Source: CAD feature listing. Evaluate the final solid. Frame: model axes, mm. A direction names the side the tool comes from. Round coordinates to 2 decimals unless told otherwise and drop trailing zeros. Order: outer loops, then holes, each group sorted by start corner. A loop starts at its lowest first (then second) coordinate and runs counter-clockwise, first axis right, second up. Notation, with made-up numbers: (70, -38) -> (114, -38) arc R19 ccw to (114, -32) -> close; hole circle Ø11 at (-21, 36.25). An arc over 180 degrees is marked (long way). Write item = value, one per line. Start each with the question number.
(1) Cut plane D-D on z = -25. Return the cut outline in (x, y).
(2) Cut plane A-A on y = 0. Return the cut outline in (x, z).
(3) Ray query, line 1 (Y direction, x = 3.3, z = 0); line 2 (Y direction, x = 3.6, z = 23); line 3 (Z direction, x = 4.2, y = -25). Return the intervals inside material, ascending.
(4) Cut plane C-C on x = 2.5. Give the number of separate pieces and of enclosed holes in the cut face, then the cut area to 3 significant figures.
(5) Contact query for flat-ended pins moving along their axis: pin 1 Ø1.5 at (x, z) = (1.5, -17.5) entering from -Y; pin 2 Ø2.5 at (x, z) = (3, 24.5) entering from +Y. Output: stop coordinate, or through.
(6) Draft query along Z for faces 5 (the face through (2, 0, -60)), 6 (the face through (2, 30, -53)), 7 (the face through (3, -33, -7.5)). Return one class per face: released by +Z, released by -Z, zero draft, split by the parting line, or undercut.
(7) Reachability of faces 1 (the face through (2, -30, 53)), 2 (the face through (2.54, -27.24, 45.96)), 3 (the face through (3, 26, -22.1)), 4 (the face through (3, -33, 7.5)) from +Z, -Z, +X, -X, +Y, -Y: full face, straight path, thin tool, end or side. Return the list, or none.
(8) Cut plane B-B on z = 0. Return the cut outline in (x, y).
from build123d import *

# Parameters (mm, degrees)
SKETCH_1_W          = 120
SKETCH_1_H          = 60
EXTRUDE_1_DEPTH     = 5
SKETCH_2_R          = 8
CUT_EXTRUDE_1_DEPTH = 5
SKETCH_3_W          = 15
SKETCH_3_H          = 5
EXTRUDE_2_DEPTH     = 5
CUT_EXTRUDE_2_DEPTH = 5
CUT_EXTRUDE_3_DEPTH = 10
FILLET_1_R          = 3
CUT_EXTRUDE_4_DEPTH = 10
FILLET_2_R          = 2


with BuildPart() as part:
    # 草图1 → 凸台-拉伸1 (new body)
    with BuildSketch(Plane(origin=(0, 0, 0), x_dir=(0, 0, -1), z_dir=(1, 0, 0))):
        Rectangle(SKETCH_1_W, SKETCH_1_H)
    extrude(amount=EXTRUDE_1_DEPTH)

    # 草图2 → 切除-拉伸1 (cut, symmetric)
    with BuildSketch(Plane(origin=(5, 0, 0), x_dir=(0, 0, -1), z_dir=(1, 0, 0))):
        Circle(SKETCH_2_R)
    extrude(amount=CUT_EXTRUDE_1_DEPTH, both=True, mode=Mode.SUBTRACT)

    # 草图3 → 凸台-拉伸2 (add)
    with BuildSketch(Plane(origin=(5, 0, 0), x_dir=(0, 0, -1), z_dir=(1, 0, 0))):
        with Locations((0, 32.5)):
            Rectangle(SKETCH_3_W, SKETCH_3_H)
        with Locations((-40, 32.5)):
            Rectangle(SKETCH_3_W, SKETCH_3_H)
        with Locations((40, 32.5)):
            Rectangle(SKETCH_3_W, SKETCH_3_H)
        with Locations((40, -32.5)):
            Rectangle(SKETCH_3_W, SKETCH_3_H)
        with Locations((-40, -32.5)):
            Rectangle(SKETCH_3_W, SKETCH_3_H)
        with Locations((0, -32.5)):
            Rectangle(SKETCH_3_W, SKETCH_3_H)
    extrude(amount=-EXTRUDE_2_DEPTH)

    # 草图4 → 切除-拉伸2 (cut)
    with BuildSketch(Plane(origin=(5, 0, 0), x_dir=(0, 0, -1), z_dir=(1, 0, 0))):
        Polygon((-22.1, 30), (-22.1, 22), (-23.5, 22), (-23.5, 15), (-16.5, 15), (-16.5, 22), (-17.9, 22), (-17.9, 30), align=None)
        Polygon((17.9, 30), (17.9, 22), (16.5, 22), (16.5, 15), (23.5, 15), (23.5, 22), (22.1, 22), (22.1, 30), align=None)
        Polygon((22.1, -30), (22.1, -22), (23.5, -22), (23.5, -15), (16.5, -15), (16.5, -22), (17.9, -22), (17.9, -30), align=None)
        Polygon((-17.9, -30), (-17.9, -22), (-16.5, -22), (-16.5, -15), (-23.5, -15), (-23.5, -22), (-22.1, -22), (-22.1, -30), align=None)
    extrude(amount=-CUT_EXTRUDE_2_DEPTH, mode=Mode.SUBTRACT)

    # 草图5 → 切除-拉伸3 (cut)
    with BuildSketch(Plane(origin=(5, 0, 0), x_dir=(0, 0, -1), z_dir=(1, 0, 0))):
        with BuildLine():
            Line((-46.321552745, 25.480053053), (-41.931231517, 9.173145635))
            ThreePointArc((-41.931231517, 9.173145635), (-40, 7.693092582), (-38.068768483, 9.173145635))
            Line((-38.068768483, 9.173145635), (-33.678447255, 25.480053053))
            ThreePointArc((-33.678447255, 25.480053053), (-34.022244696, 27.216574311), (-35.609678772, 28))
            Line((-35.609678772, 28), (-44.390321228, 28))
            ThreePointArc((-44.390321228, 28), (-45.977755304, 27.216574311), (-46.321552745, 25.480053053))
        make_face()
        with BuildLine():
            Line((-49.120413153, 22.331136171), (-41.994161638, 2.733944505))
            ThreePointArc((-41.994161638, 2.733944505), (-41.512509026, 0), (-41.994161638, -2.733944505))
            Line((-41.994161638, -2.733944505), (-49.120413153, -22.331136171))
            ThreePointArc((-49.120413153, -22.331136171), (-51.347005984, -23.617316729), (-53, -21.647650045))
            Line((-53, -21.647650045), (-53, 21.647650045))
            ThreePointArc((-53, 21.647650045), (-51.347005984, 23.617316729), (-49.120413153, 22.331136171))
        make_face()
        with BuildLine():
            Line((-38.068768483, -9.173145635), (-33.678447255, -25.480053053))
            ThreePointArc((-33.678447255, -25.480053053), (-34.022244696, -27.216574311), (-35.609678772, -28))
            Line((-35.609678772, -28), (-44.390321228, -28))
            ThreePointArc((-44.390321228, -28), (-45.977755304, -27.216574311), (-46.321552745, -25.480053053))
            Line((-46.321552745, -25.480053053), (-41.931231517, -9.173145635))
            ThreePointArc((-41.931231517, -9.173145635), (-40, -7.693092582), (-38.068768483, -9.173145635))
        make_face()
        with BuildLine():
            Line((-38.005838362, -2.733944505), (-30.879586847, -22.331136171))
            ThreePointArc((-30.879586847, -22.331136171), (-28.652994016, -23.617316729), (-27, -21.647650045))
            Line((-27, -21.647650045), (-27, 21.647650045))
            ThreePointArc((-27, 21.647650045), (-28.652994016, 23.617316729), (-30.879586847, 22.331136171))
            Line((-30.879586847, 22.331136171), (-38.005838362, 2.733944505))
            ThreePointArc((-38.005838362, 2.733944505), (-38.487490974, 0), (-38.005838362, -2.733944505))
        make_face()
        with BuildLine():
            Line((27, -21.647650045), (27, 21.647650045))
            ThreePointArc((27, 21.647650045), (28.652994016, 23.617316729), (30.879586847, 22.331136171))
            Line((30.879586847, 22.331136171), (38.005838362, 2.733944505))
            ThreePointArc((38.005838362, 2.733944505), (38.487490974, 0), (38.005838362, -2.733944505))
            Line((38.005838362, -2.733944505), (30.879586847, -22.331136171))
            ThreePointArc((30.879586847, -22.331136171), (28.652994016, -23.617316729), (27, -21.647650045))
        make_face()
        with BuildLine():
            Line((35.609678772, -28), (44.390321228, -28))
            ThreePointArc((44.390321228, -28), (45.977755304, -27.216574311), (46.321552745, -25.480053053))
            Line((46.321552745, -25.480053053), (41.931231517, -9.173145635))
            ThreePointArc((41.931231517, -9.173145635), (40, -7.693092582), (38.068768483, -9.173145635))
            Line((38.068768483, -9.173145635), (33.678447255, -25.480053053))
            ThreePointArc((33.678447255, -25.480053053), (34.022244696, -27.216574311), (35.609678772, -28))
        make_face()
        with BuildLine():
            Line((53, -21.647650045), (53, 21.647650045))
            ThreePointArc((53, 21.647650045), (51.347005984, 23.617316729), (49.120413153, 22.331136171))
            Line((49.120413153, 22.331136171), (41.994161638, 2.733944505))
            ThreePointArc((41.994161638, 2.733944505), (41.512509026, 0), (41.994161638, -2.733944505))
            Line((41.994161638, -2.733944505), (49.120413153, -22.331136171))
            ThreePointArc((49.120413153, -22.331136171), (51.347005984, -23.617316729), (53, -21.647650045))
        make_face()
        with BuildLine():
            Line((35.609678772, 28), (44.390321228, 28))
            ThreePointArc((44.390321228, 28), (45.977755304, 27.216574311), (46.321552745, 25.480053053))
            Line((46.321552745, 25.480053053), (41.931231517, 9.173145635))
            ThreePointArc((41.931231517, 9.173145635), (40, 7.693092582), (38.068768483, 9.173145635))
            Line((38.068768483, 9.173145635), (33.678447255, 25.480053053))
            ThreePointArc((33.678447255, 25.480053053), (34.022244696, 27.216574311), (35.609678772, 28))
        make_face()
    extrude(amount=-CUT_EXTRUDE_3_DEPTH, mode=Mode.SUBTRACT)

    # 圆角1
    fillet_1_edges = [part.edges().sort_by_distance(p)[0] for p in [
        (2.5, 30, 60),
        (2.5, 30, -60),
        (2.5, -30, -60),
        (2.5, -30, 60),
    ]]
    fillet(fillet_1_edges, radius=FILLET_1_R)

    # 草图6 → 切除-拉伸4 (cut)
    with BuildSketch(Plane(origin=(5, 0, 0), x_dir=(0, 0, -1), z_dir=(1, 0, 0))):
        with BuildLine():
            Line((-49.5, 30), (-47.5, 30))
            ThreePointArc((-47.5, 30), (-48.5, 29), (-49.5, 30))
        make_face()
        with BuildLine():
            Line((-32.5, 30), (-30.5, 30))
            ThreePointArc((-30.5, 30), (-31.5, 29), (-32.5, 30))
        make_face()
        with BuildLine():
            Line((-9.5, 30), (-7.5, 30))
            ThreePointArc((-7.5, 30), (-8.5, 29), (-9.5, 30))
        make_face()
        with BuildLine():
            Line((7.5, 30), (9.5, 30))
            ThreePointArc((9.5, 30), (8.5, 29), (7.5, 30))
        make_face()
        with BuildLine():
            Line((30.5, 30), (32.5, 30))
            ThreePointArc((32.5, 30), (31.5, 29), (30.5, 30))
        make_face()
        with BuildLine():
            Line((47.5, 30), (49.5, 30))
            ThreePointArc((49.5, 30), (48.5, 29), (47.5, 30))
        make_face()
        with BuildLine():
            Line((47.5, -30), (49.5, -30))
            ThreePointArc((49.5, -30), (48.5, -29), (47.5, -30))
        make_face()
        with BuildLine():
            Line((30.5, -30), (32.5, -30))
            ThreePointArc((32.5, -30), (31.5, -29), (30.5, -30))
        make_face()
        with BuildLine():
            Line((7.5, -30), (9.5, -30))
            ThreePointArc((9.5, -30), (8.5, -29), (7.5, -30))
        make_face()
        with BuildLine():
            Line((-9.5, -30), (-7.5, -30))
            ThreePointArc((-7.5, -30), (-8.5, -29), (-9.5, -30))
        make_face()
        with BuildLine():
            Line((-32.5, -30), (-30.5, -30))
            ThreePointArc((-30.5, -30), (-31.5, -29), (-32.5, -30))
        make_face()
        with BuildLine():
            Line((-49.5, -30), (-47.5, -30))
            ThreePointArc((-47.5, -30), (-48.5, -29), (-49.5, -30))
        make_face()
    extrude(amount=-CUT_EXTRUDE_4_DEPTH, mode=Mode.SUBTRACT)

    # 圆角2
    fillet_2_edges = [part.edges().sort_by_distance(p)[0] for p in [
        (2.5, -15, 23.5),
        (2.5, -15, 16.5),
        (2.5, -15, -16.5),
        (2.5, -15, -23.5),
        (2.5, 15, -23.5),
        (2.5, 15, -16.5),
        (2.5, 15, 16.5),
        (2.5, 15, 23.5),
    ]]
    fillet(fillet_2_edges, radius=FILLET_2_R)


solid = part.part
Evaluation:
q1.outline = (0, -30) -> (5, -30) -> (5, 30) -> (0, 30) -> close
q2.outline = (0, -60) -> (5, -60) -> (5, -53) -> (0, -53) -> close; (0, -41.51) -> (5, -41.51) -> (5, -38.49) -> (0, -38.49) -> close; (0, -27) -> (5, -27) -> (5, -8) -> (0, -8) -> close; (0, 8) -> (5, 8) -> (5, 27) -> (0, 27) -> close; (0, 38.49) -> (5, 38.49) -> (5, 41.51) -> (0, 41.51) -> close; (0, 53) -> (5, 53) -> (5, 60) -> (0, 60) -> close
q3.line_1 = -35 to -8, 8 to 35
q3.line_2 = -30 to -22, -15.68 to 15.68, 22 to 30
q3.line_3 = -60 to -46.19, -33.81 to -22.1, -17.9 to 17.9, 22.1 to 33.81, 46.19 to 60
q4.separate_pieces = 1
q4.enclosed_holes = 9
q4.area = 4,980 mm^2
q5.pin_1 = -30
q5.pin_2 = 30
q6.face_5 = released by -Z
q6.face_6 = zero draft
q6.face_7 = undercut
q7.face_1 = +Z, +X, -X, -Y
q7.face_2 = +X, -X
q7.face_3 = +X, -X, +Y
q7.face_4 = +X, -X, -Y
q8.outline = (0, -35) -> (5, -35) -> (5, -8) -> (0, -8) -> close; (0, 8) -> (5, 8) -> (5, 35) -> (0, 35) -> close
